```python
from build123d import *

# Parameters (mm, degrees)
SKETCH1_W           = 96.613496933
SKETCH1_H           = 50.8
BOSS_EXTRUDE1_DEPTH = 21
SKETCH4_R           = 14.134180844
BOSS_EXTRUDE2_DEPTH = 21


with BuildPart() as part:
    # Sketch1 → Boss-Extrude1 (new body)
    with BuildSketch(Plane.XY):
        with Locations((-0.623312883, 1.86993865)):
            Rectangle(SKETCH1_W, SKETCH1_H)
    extrude(amount=BOSS_EXTRUDE1_DEPTH)

    # Sketch4 → Boss-Extrude2 (add)
    with BuildSketch(Plane.XY.offset(21)):
        Circle(SKETCH4_R)
    extrude(amount=BOSS_EXTRUDE2_DEPTH)


solid = part.part
```
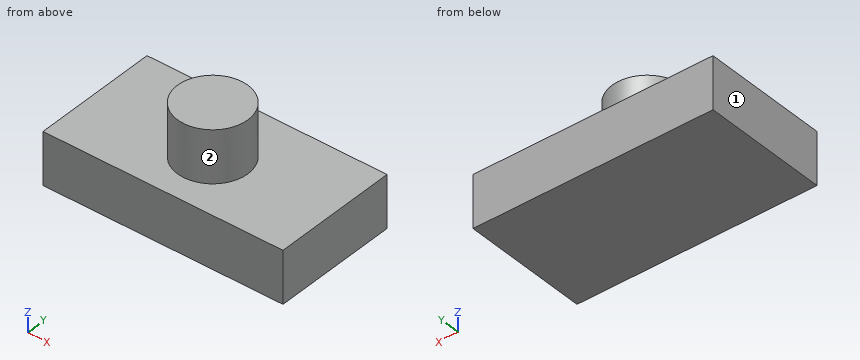
Geometry: final body of the model. Coordinates: model frame, mm. Face numbers are marked on the shaded views. A direction names the side the tool comes from. Coordinates: 2 decimals unless noted, no trailing zeros. Order: outer loops, then holes, each group sorted by start corner. A loop starts at its lowest first (then second) coordinate and runs counter-clockwise, first axis right, second up.
Item 1: Material intervals for line 1 along Z through (x, y) = (-3.5, 23); line 2 along Y through (x, z) = (6, 27); line 3 along X through (y, z) = (-2.5, 36), sorted ascending.
Answer:
line 1: z = 0 to 21
line 2: y = -12.8 to 12.8
line 3: x = -13.91 to 13.91
Item 2: Section query C-C (z = 39.5). Output: boundary loops of the cut face in (x, y).
Answer:
outline: circle Ø28.27 at (0, 0)
Item 3: Section query D-D (y = 23). Output: boundary loops of the cut face in (x, z).
Answer:
outline: (-48.93, 0) - (47.68, 0) - (47.68, 21) - (-48.93, 21) - close
Item 4: Section query A-A (y = 0). Output: boundary loops of the cut face in (x, z).
Answer:
outline: (-48.93, 0) - (47.68, 0) - (47.68, 21) - (14.13, 21) - (14.13, 42) - (-14.13, 42) - (-14.13, 21) - (-48.93, 21) - close
Item 5: Section query B-B (x = 4). Output: boundary loops of the cut face in (y, z), then the cut area to 3 significant figures.
Answer:
outline: (-23.53, 0) - (27.27, 0) - (27.27, 21) - (13.56, 21) - (13.56, 42) - (-13.56, 42) - (-13.56, 21) - (-23.53, 21) - close
area: 1,640 mm2
Item 6: Contact query for a flat-ended pin moving along its axis: P1, Ø4, axis at x = 37, y = 20, coming from the +Z side. Output: stop coordinate, or through.
Answer:
P1: stops at z = 21
Item 7: Access query for the marked faces 1 and 2. Directions: +Z, -Z, +X, -X, +Y, -Y. A direction counts if a zero-diameter tool reaches every point of the face in a straight line with its end or side. Return the directions, or none.
Answer:
face 1: +Z, -Z, -X, +Y, -Y
face 2: +Z
